Autodesk Inventor part; units mm, degrees
ref_plane "YZ Plane" through (0, 0, 0) normal (1, 0, 0) x (0, 1, 0)
ref_plane "XZ Plane" through (0, 0, 0) normal (0, 1, 0) x (-1, 0, 0)
ref_plane "XY Plane" through (0, 0, 0) normal (0, 0, 1) x (1, 0, 0)
sketch "Skizze1" plane through (0, 0, 0) normal (0, 0, 1) x (1, 0, 0)
  circle A0 centre (0, 0) radius 8
  dimension "d0" = 16
extrude "Extrusion1" add sketch "Skizze1" along normal blind 3
chamfer "Fase1" distance 1 angle 45 1 edges at (-8, 0, 3)
hole "Bohrung1" at (0, 0, 0) direction (0, 0, 1) diameter 3.4 depth 8 tip angle 118
properties part number "Capstondisc_v2_Anschlagscheibe" material "Aluminium 6061"
The listing builds one solid part. Answer for the finished solid, in the listing's coordinates (mm). Round coordinates to 2 decimals unless told otherwise and drop trailing zeros. Loops run counter-clockwise (first coordinate to the right, second up) from the corner with the lowest first, then second, coordinate; pieces in that order, holes last.
Q1. For a pull along X with two mould halves and no side action, classify faces 1 (the face through (1.66, -0.37, 1.52)), 2 (the face through (-1.73, 7.81, 0.99)), 3 (the face through (1.5, -1.5, 3)) as released by +X, released by -X, zero draft, split by the parting line, or undercut.
Q2. Section A-A, the plane x = 0 is taken. Determine the outline of the cut face in (y, z).
Q3. Given pin 1 Ø6 at (x, y) = (4.5, 1.5) entering from -Z, flat-ended and moving along its own axis, determine where the tip first touches the part or whether it passes through.
Q4. Section C-C, the plane z = 1.3 is taken. Determine the outline of the cut face in (x, y).
Q5. Find the intervals of material crossed by line 1 (Y direction, x = 0, z = 0.7); line 2 (X direction, y = 0, z = 2.05); line 3 (X direction, y = 0.5, z = 2.3), in increasing order.
Completed:
1. face 1: undercut
1. face 2: split by the parting line
1. face 3: zero draft
2. outline: (-8, 0) - (-1.7, 0) - (-1.7, 3) - (-7, 3) - (-8, 2) - close; (1.7, 0) - (8, 0) - (8, 2) - (7, 3) - (1.7, 3) - close
3. pin 1: stops at z = 0
4. outline: circle Ø16 at (0, 0); hole circle Ø3.4 at (0, 0)
5. line 1: y = -8 to -1.7, 1.7 to 8
5. line 2: x = -7.95 to -1.7, 1.7 to 7.95
5. line 3: x = -7.68 to -1.62, 1.62 to 7.68
